```python
from build123d import *

# Parameters (mm, degrees)
F0_W     = 5.08
F0_H     = 25.4
F0_W_2   = 2.54
F0_W_3   = 3.81
F1_DEPTH = 40
F3_W     = 2
F3_H     = 11.758205078
F3_W_2   = 1.5
F3_W_3   = 1
F3_W_4   = 0.4
F3_W_5   = 0.5
F4_DEPTH = 12.5


with BuildPart() as f1:
    # F0 (on Front) → F1 (new body)
    with BuildSketch(Plane.XZ):
        Polygon((-39.5374095005, -17.8057016992), (-44.6174095005, -17.8057016992), (-44.6174095005, -22.8857016992), (56.9825904995, -22.8857016992), (56.9825904995, -17.8057016992), (51.9025904995, -17.8057016992), (40.6538585508, -17.8057016992), (38.1138585508, -17.8057016992), (25.9218535846, -17.8057016992), (22.1118535846, -17.8057016992), (8.1349273361, -17.8057016992), (3.0549273361, -17.8057016992), (-17.8261825508, -17.8057016992), (-20.3661825508, -17.8057016992), (-27.4666358256, -17.8057016992), (-31.2766358256, -17.8057016992), align=None)
        with Locations((54.4425904995, -5.1057016992)):
            Rectangle(F0_W, F0_H)
        with Locations((39.3838585508, -5.1057016992)):
            Rectangle(F0_W_2, F0_H)
        with Locations((24.0168535846, -5.1057016992)):
            Rectangle(F0_W_3, F0_H)
        with Locations((5.5949273361, -5.1057016992)):
            Rectangle(F0_W, F0_H)
        with Locations((-29.3716358256, -5.1057016992)):
            Rectangle(F0_W_3, F0_H)
        with Locations((-42.0774095005, -5.1057016992)):
            Rectangle(F0_W, F0_H)
        with Locations((-19.0961825508, -5.1057016992)):
            Rectangle(F0_W_2, F0_H)
    extrude(amount=F1_DEPTH)


with BuildPart() as f4:
    # F3 (on Front) → F4 (new body, symmetric)
    with BuildSketch(Plane.XZ):
        with Locations((-14.0355701865, -5.879102539)):
            Rectangle(F3_W, F3_H)
        Polygon((-13.0355701865, -11.758205078), (-15.0355701865, -11.758205078), (-15.0355701865, -14.758205078), (-0.0355701865, -14.758205078), (-0.0355701865, -11.758205078), (-0.0385628735, -11.758205078), (-0.4385628735, -11.758205078), (-1.1385628735, -11.758205078), (-1.5385628735, -11.758205078), (-2.2385628735, -11.758205078), (-2.6385628735, -11.758205078), (-4.3532104, -11.758205078), (-4.8532104, -11.758205078), (-5.4532104, -11.758205078), (-5.9532104, -11.758205078), (-6.5532104, -11.758205078), (-7.0532104, -11.758205078), (-7.870703689, -11.758205078), (-8.870703689, -11.758205078), (-10.0352638757, -11.758205078), (-11.5352638757, -11.758205078), align=None)
        with Locations((-10.7852638757, -5.879102539)):
            Rectangle(F3_W_2, F3_H)
        with Locations((-8.370703689, -5.879102539)):
            Rectangle(F3_W_3, F3_H)
        with Locations((-0.2385628735, -5.879102539)):
            Rectangle(F3_W_4, F3_H)
        with Locations((-6.8032104, -5.879102539)):
            Rectangle(F3_W_5, F3_H)
        with Locations((-1.3385628735, -5.879102539)):
            Rectangle(F3_W_4, F3_H)
        with Locations((-5.7032104, -5.879102539)):
            Rectangle(F3_W_5, F3_H)
        with Locations((-2.4385628735, -5.879102539)):
            Rectangle(F3_W_4, F3_H)
        with Locations((-4.6032104, -5.879102539)):
            Rectangle(F3_W_5, F3_H)
    extrude(amount=F4_DEPTH, both=True)


solid = f4.part
```
Work out the finished part from the listing and answer in its coordinate system (mm). A direction names the side the tool comes from. Give positions to 0.01 mm unless a question says otherwise; leave off trailing zeros. Order: outer loops, then holes, each group sorted by start corner. A loop starts at its lowest first (then second) coordinate and runs counter-clockwise, first axis right, second up. Notation, with made-up numbers: (50.25, 20) -> (84.25, 20) arc R13 cw to (84.25, 26) -> close; hole circle Ø1 at (-0.5, 52). An arc over 180 degrees is marked (long way). Answer as CSV lines item,"result". Start each with the question number.
(1) For a pull along X with two mould halves and no side action, classify faces 3 (the flat face through (-15.036, 0, -7)), 4 (the flat face through (-9.4, -0.2, -11.758)), 5 (the flat face through (-11, -12.5, -11)) as released by +X, released by -X, zero draft, split by the parting line, or undercut.
(2) Section A-A, the plane z = -1.25 is taken. Give the number of separate pieces and of enclosed holes in the cut face, plus the area to 3 significant figures.
(3) Which of the six approach directions +Z, -Z, +X, -X, +Y, -Y give full straight-line access (tool end or side, diameter ignored) to faces 1 (the flat face through (-2.239, 0, -6)), 2 (the flat face through (-8.4, -0.2, 0))?
(4) Consider line 1 along Z through (x, y) = (-4.25, 5.5). Determine where the line is inside the solid, lowest interval first.
(5) Each of these flat-tipped pins is pushed along its axis until it touches: pin 1 Ø0.9 at (x, y) = (-3.5, -3.5) entering from +Z; pin 2 Ø0.9 at (x, y) = (-7.5, -4) entering from +Z; pin 3 Ø3.5 at (y, z) = (1.5, -4) entering from +X. Where does it stop, or does it pass through?
(6) Section B-B, the plane x = -9.25 is taken. Write down the section's boundary in (y, z), plus the area to 3 significant figures.
Entries:
1,face 3,"released by -X"
1,face 4,"undercut"
1,face 5,"zero draft"
2,separate pieces,"9"
2,enclosed holes,"0"
2,area,"180 mm²"
3,face 1,"+Z, +Y, -Y"
3,face 2,"+Z, +X, -X, +Y, -Y"
4,line 1,"-14.76 to -11.76"
5,pin 1,"z = -11.76"
5,pin 2,"z = 0"
5,pin 3,"x = -0.04"
6,outline,"(-12.5, -14.76) -> (12.5, -14.76) -> (12.5, -11.76) -> (-12.5, -11.76) -> close"
6,area,"75.0 mm²"
